Job drawing, mm, ordinate dimensions from the low corner. One solid piece. A direction names the side the tool comes from. Round coordinates to 2 decimals unless told otherwise and drop trailing zeros. Loops run counter-clockwise (first coordinate to the right, second up) from the corner with the lowest first, then second, coordinate; pieces in that order, holes last. Notation, with made-up numbers: (1, -27.5) - (30, -27.5) arc R7 cw to (30, -18.5) - close; hole circle Ø10 at (81.5, -20). An arc over 180 degrees is marked (long way). Answer as CSV lines item,"result". Start each with the question number.
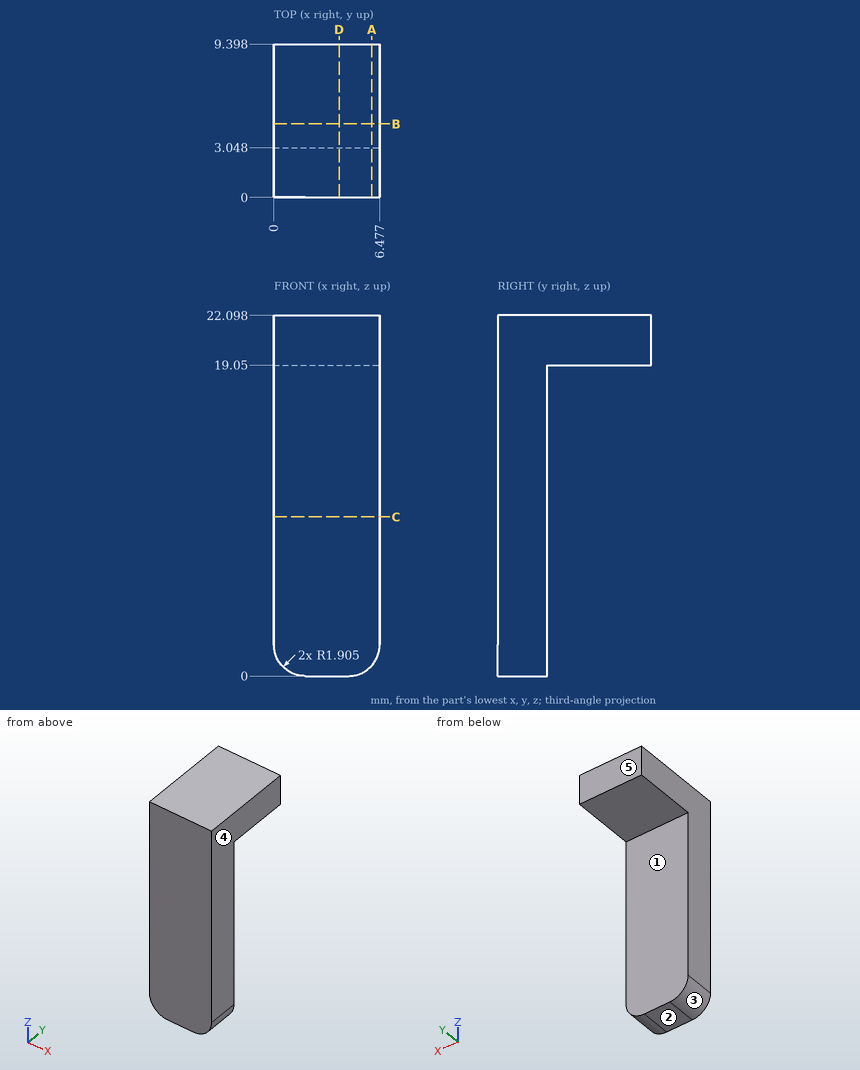
Q1. Pin check, flat tips, straight feed: pin 1 Ø2 at (x, z) = (4, 8.5) entering from +Y; pin 2 Ø3 at (x, y) = (2, 5.5) entering from -Z. Stop position of each tip, or through.
Q2. Band-saw the part on A-A, the plane x = 6. List the corners of the cut face in (y, z), then the cut area to 3 significant figures.
Q3. Two-plate mould, pull along X, no slides. Class the marked faces 3, 4 and 5: released by +X, released by -X, zero draft, split by the parting line, or undercut.
Q4. Tool access for the marked faces 1 and 2: list every direction of +Z, -Z, +X, -X, +Y, -Y with a clear straight run to the whole face (end or side of a thin tool).
Q5. Band-saw the part on C-C, the plane z = 9.75. List the corners of the cut face in (x, y), then the cut area to 3 significant figures.
Q6. Wall check: probe 1 along Z at (x, y) = (3.5, 8); probe 2 along Y at (x, z) = (0.75, 6.5); probe 3 along Z at (x, y) = (1, 2.5). Give the ranges that are in metal, low to high. Write a range as [from, to].
Q7. Band-saw the part on D-D, the plane x = 4. List the corners of the cut face in (y, z).
Q8. Band-saw the part on B-B, the plane y = 4.5. List the corners of the cut face in (x, z), then the cut area to 3 significant figures.
Reported:
1,pin 1,"stops at y = 3.05"
1,pin 2,"stops at z = 19.05"
2,outline,"(0, 0.64) - (3.05, 0.64) - (3.05, 19.05) - (9.4, 19.05) - (9.4, 22.1) - (0, 22.1) - close"
2,area,"84.7 mm2"
3,face 3,"released by -X"
3,face 4,"released by +X"
3,face 5,"zero draft"
4,face 1,"-Z, +X, -X, +Y"
4,face 2,"-Z, +X, -X, +Y, -Y"
5,outline,"(0, 0) - (6.48, 0) - (6.48, 3.05) - (0, 3.05) - close"
5,area,"19.7 mm2"
6,probe 1,"z = [19.05, 22.1]"
6,probe 2,"y = [0, 3.05]"
6,probe 3,"z = [0.23, 22.1]"
7,outline,"(0, 0) - (3.05, 0) - (3.05, 19.05) - (9.4, 19.05) - (9.4, 22.1) - (0, 22.1) - close"
8,outline,"(0, 19.05) - (6.48, 19.05) - (6.48, 22.1) - (0, 22.1) - close"
8,area,"19.7 mm2"
